Check sheet for the modelled part. Datum: model origin and axes. Units: mm. A direction names the side the tool comes from. Round coordinates to 2 decimals unless told otherwise and drop trailing zeros. Order: outer loops, then holes, each group sorted by start corner. A loop starts at its lowest first (then second) coordinate and runs counter-clockwise, first axis right, second up.
(1) Sectioned sample at A-A, the plane x = 31. Enter the section's corners in (y, z), and give its area (3 significant figures).
(2) Depth check by flat-ended pin: pin 1 (3 mm diameter, centred on x = -15.5, y = 1.5, fed in from +Z); pin 2 (6 mm diameter, centred on x = 0, y = 4.5, fed in from +Z); pin 3 (2 mm diameter, centred on x = 32, y = 1.5, fed in from -Z). Enter the tip coordinate at first touch or a pass-through.
(3) Sectioned sample at B-B, the plane y = 4.5. Enter the section's corners in (x, z).
(4) Mould release check, pull along Z, two halves, no side actions. Record for faces 1 (the cylindrical face through (-0.35, 4.93, 93.99)), 2 (the cylindrical face through (-16.05, 4.93, 73.295)), 3 (the cylindrical face through (44.93, 4.93, 89.37)), 4 (the flat face through (17.2, 4.9, 32.5)): released by +Z, released by -Z, zero draft, split by the parting line, or undercut.
(5) Sectioned sample at D-D, the plane x = 15. Enter the section's corners in (y, z), and give its area (3 significant figures).
(6) Thickness scan on probe 1 along X at (y, z) = (7.25, 88); probe 2 along Z at (x, y) = (-31, 6); probe 3 along X at (y, z) = (3, 84). Record the ranges inside material, lowest first.
(7) Tool access check on faces 5 (the flat face through (-17.33, 4.93, 31.61)), 6 (the cylindrical face through (31.242, 4.93, 82.505)). Record the directions out of +Z, -Z, +X, -X, +Y, -Y that give a thin tool (end or side, any length) a straight path to the whole face; none if there is none.
(8) Sectioned sample at C-C, the plane z = 91.5. Enter the section's corners in (x, y), and give its area (3 significant figures).
```python
from build123d import *

# Parameters (mm, degrees)
SKETCH1_R           = 10
SKETCH1_R_2         = 5.5
BOSS_EXTRUDE1_DEPTH = 10


with BuildPart() as part:
    # Sketch1 → Boss-Extrude1 (new body)
    with BuildSketch(Plane(origin=(0, 0, 0), x_dir=(1, 0, 0), z_dir=(0, 1, 0))):
        with BuildLine():
            Line((-22, 0), (-12.527017524, -64.124804454))
            ThreePointArc((-12.527017524, -64.124804454), (-16.163432373, -73.387478219), (-25.994798684, -74.925293128))
            ThreePointArc((-25.994798684, -74.925293128), (-44.965677172, -88.979725021), (-24.218363132, -100.247832518))
            ThreePointArc((-24.218363132, -100.247832518), (0.000559759, -93.990091526), (24.21978519, -100.246661496))
            ThreePointArc((24.21978519, -100.246661496), (44.96401141, -88.978987225), (25.994886362, -74.927094121))
            ThreePointArc((25.994886362, -74.927094121), (16.163301714, -73.389548338), (12.526730263, -64.126748988))
            Line((12.526730263, -64.126748988), (22, 0))
            ThreePointArc((22, 0), (0, 22), (-22, 0))
        make_face()
        with Locations(Location((0, 0, 0), (0, 0, 270))):
            Circle(SKETCH1_R, mode=Mode.SUBTRACT)
        with Locations(Location((31, -88, 0), (0, 0, 270))):
            Circle(SKETCH1_R_2, mode=Mode.SUBTRACT)
        with Locations(Location((-31, -88, 0), (0, 0, 90))):
            Circle(SKETCH1_R_2, mode=Mode.SUBTRACT)
    extrude(amount=BOSS_EXTRUDE1_DEPTH)


solid = part.part
```
Derived:
1. outline: (0, 74) - (10, 74) - (10, 82.5) - (0, 82.5) - close; (0, 93.5) - (10, 93.5) - (10, 102) - (0, 102) - close
1. area: 170 mm2
2. pin 1: stops at z = 96.97
2. pin 2: stops at z = 94.08
2. pin 3: stops at z = 74
3. outline: (-25.99, 74.93) arc R10 cw to (-12.53, 64.12) - (-22, 0) arc R22 ccw to (22, 0) - (12.53, 64.13) arc R10 cw to (25.99, 74.93) arc R14 ccw (long way) to (24.22, 100.25) arc R50 cw to (-24.22, 100.25) arc R14 ccw (long way) to start; hole circle Ø11 at (-31, 88); hole circle Ø20 at (0, 0); hole circle Ø11 at (31, 88)
4. face 1: released by +Z
4. face 2: undercut
4. face 3: split by the parting line
4. face 4: undercut
5. outline: (0, -16.09) - (10, -16.09) - (10, 47.38) - (0, 47.38) - close; (0, 72.29) - (10, 72.29) - (10, 96.29) - (0, 96.29) - close
5. area: 875 mm2
6. probe 1: x = -45 to -36.5, -25.5 to 25.5, 36.5 to 45
6. probe 2: z = 74 to 82.5, 93.5 to 102
6. probe 3: x = -44.42 to -34.77, -27.23 to 27.23, 34.77 to 44.41
7. face 5: -X, +Y, -Y
7. face 6: +Y, -Y
8. outline: (-44.56, 0) - (-35.24, 0) - (-35.24, 10) - (-44.56, 10) - close; (-26.76, 0) - (26.76, 0) - (26.76, 10) - (-26.76, 10) - close; (35.24, 0) - (44.55, 0) - (44.55, 10) - (35.24, 10) - close
8. area: 721 mm2
